Here's how the part is built. I have some questions about the finished solid (model axes, mm). A direction names the side the tool comes from. Coordinates: 2 decimals unless noted, no trailing zeros. Write each loop counter-clockwise with the first axis right and the second up, starting at its lowest first coordinate (ties: lowest second). Pieces come first, ordered by that corner, then holes. Notation, with made-up numbers: M 80.25,67.5 L 85.25,67.5 A18 cw 85.25,99.5 Z; hole C -6.5,19.5 d2. An arc over 180 degrees is marked long. Use a Markdown table: item, result.
```python
from build123d import *

# Parameters (mm, degrees)
F0_R          = 37.5
F1_DEPTH      = 25
F2_R          = 22.5
F3_DEPTH      = 80
F3_DEPTH_BACK = 80
F5_START      = 25
F4_R          = 42.5
F5_DEPTH      = 25


with BuildPart() as f1:
    # F0 (on Top) → F1 (new body)
    with BuildSketch(Plane.XY):
        Circle(F0_R)
    extrude(amount=F1_DEPTH)

    # F2 (on face) → F3 (join, two sides)
    with BuildSketch(Plane.XY.offset(25)) as f3_sk:
        Circle(F2_R)
    extrude(amount=-F3_DEPTH)
    extrude(f3_sk.sketch, amount=F3_DEPTH_BACK)

    # F4 (on face) → F5 (join)
    with BuildSketch(Plane.XY.offset(25).offset(F5_START)):
        Circle(F4_R)
    extrude(amount=F5_DEPTH)


solid = f1.part
```
1. Suppose I cut it at A-A on y = 0. Write out the boundary of the cut face in (x, z), and give its area (3 significant figures).
Answers follow:
| item | result |
|---|---|
| outline | M -42.5,50 L -22.5,50 L -22.5,25 L -37.5,25 L -37.5,0 L -22.5,0 L -22.5,-55 L 22.5,-55 L 22.5,0 L 37.5,0 L 37.5,25 L 22.5,25 L 22.5,50 L 42.5,50 L 42.5,75 L 22.5,75 L 22.5,105 L -22.5,105 L -22.5,75 L -42.5,75 Z |
| area | 8,950 mm2 |
2. Will these pins go through, and if not, where does the flat tip stop? pin 1 Ø12 at (y, z) = (15.5, -10.5) entering from -X; pin 2 Ø10 at (y, z) = (-23.5, 2.5) entering from -X; pin 3 Ø6 at (x, z) = (1.5, 54) entering from +Y.
Answers follow:
| item | result |
|---|---|
| pin 1 | stops at x = -20.4 |
| pin 2 | stops at x = -32.62 |
| pin 3 | stops at y = 42.5 |
3. I need wall thicknesses on probe 1 along Z at (x, y) = (10.5, -20.5); probe 2 along Y at (x, z) = (-4.5, 64); probe 3 along Y at (x, z) = (-8, 12.5). Which ranges of each line are inside material? Lowest first, please.
Answers follow:
| item | result |
|---|---|
| probe 1 | z = 0 to 25, 50 to 75 |
| probe 2 | y = -42.26 to 42.26 |
| probe 3 | y = -36.64 to 36.64 |
4. Suppose I cut it at C-C on x = -24.5. Write out the boundary of the cut face in (y, z), and give its area (3 significant figures).
Answers follow:
| item | result |
|---|---|
| outline | M -34.73,50 L 34.73,50 L 34.73,75 L -34.73,75 Z; M -28.39,0 L 28.39,0 L 28.39,25 L -28.39,25 Z |
| area | 3,160 mm2 |
5. Suppose I cut it at D-D on z = 73. Write out the boundary of the cut face in (x, y).
Answers follow:
| item | result |
|---|---|
| outline | C 0,0 d85 |
6. Which directions (+Z, -Z, +X, -X, +Y, -Y) give clear straight access to the entire face, cutting with the end or side of a thin tool? Please do faces 1 (the face through (10.382, -19.961, 37.325)), 2 (the face through (0, 0, -55)), 3 (the face through (16.1, -16.1, 0)), 4 (the face through (10.382, -19.961, 89.79)).
Answers follow:
| item | result |
|---|---|
| face 1 | none |
| face 2 | -Z, +X, -X, +Y, -Y |
| face 3 | -Z |
| face 4 | +Z |
